Design review of the part built by this model. Coordinates are the model's own, in mm. A direction names the side the tool comes from. Coordinates: 2 decimals unless noted, no trailing zeros. Order: outer loops, then holes, each group sorted by start corner. A loop starts at its lowest first (then second) coordinate and runs counter-clockwise, first axis right, second up.
from build123d import *

# Parameters (mm, degrees)
SKETCH1_W           = 30.2
SKETCH1_H           = 14.75
SKETCH1_W_2         = 25.2
SKETCH1_H_2         = 9.75
BOSS_EXTRUDE1_DEPTH = 20
SKETCH2_W           = 30.2
SKETCH2_H           = 14.75
BOSS_EXTRUDE2_DEPTH = 2.5
SKETCH3_W           = 14.2
SKETCH3_H           = 17.5
CUT_EXTRUDE1_DEPTH  = 2.5
FILLET1_R           = 2.5
FILLET2_R           = 2.5
FILLET3_START       = -8
FILLET3_DEPTH       = 16
FILLET3_START_2     = 4.875
FILLET3_2_DEPTH     = 3.125
FILLET3_3_DEPTH     = 2.5


with BuildPart() as part:
    # Sketch1 → Boss-Extrude1 (new body)
    with BuildSketch(Plane(origin=(0, 0, 0), x_dir=(1, 0, 0), z_dir=(0, 1, 0))):
        Rectangle(SKETCH1_W, SKETCH1_H)
        Rectangle(SKETCH1_W_2, SKETCH1_H_2, mode=Mode.SUBTRACT)
    extrude(amount=BOSS_EXTRUDE1_DEPTH)

    # Sketch2 → Boss-Extrude2 (add)
    with BuildSketch(Plane(origin=(0, 20, 0), x_dir=(1, 0, 0), z_dir=(0, 1, 0))):
        Rectangle(SKETCH2_W, SKETCH2_H)
    extrude(amount=BOSS_EXTRUDE2_DEPTH)

    # Sketch3 → Cut-Extrude1 (cut)
    with BuildSketch(Plane.XY.offset(7.375)):
        with Locations((0, 8.75)):
            Rectangle(SKETCH3_W, SKETCH3_H)
    extrude(amount=-CUT_EXTRUDE1_DEPTH, mode=Mode.SUBTRACT)

    # Fillet1
    fillet1_edges = [part.edges().sort_by_distance(p)[0] for p in [
        (-15.1, 22.5, 0),
        (15.1, 22.5, 0),
    ]]
    fillet(fillet1_edges, radius=FILLET1_R)

    # Fillet2
    fillet2_edges = [part.edges().sort_by_distance(p)[0] for p in [
        (12.6, 20, 0),
        (-12.6, 20, 0),
    ]]
    fillet(fillet2_edges, radius=FILLET2_R)

    # Fillet3: read off the stored shape, not the designer's step
    # Fillet3 outline → Fillet3 (cut)
    with BuildSketch(Plane.XY.offset(FILLET3_START)):
        with BuildLine():
            Line((-15.1, 0), (-12.6, 0))
            ThreePointArc((-12.6, 0), (-14.367766953, 0.732233047), (-15.1, 2.5))
            Line((-15.1, 2.5), (-15.1, 0))
        make_face()
        with BuildLine():
            ThreePointArc((15.1, 2.5), (14.367766953, 0.732233047), (12.6, 0))
            Line((12.6, 0), (15.1, 0))
            Line((15.1, 0), (15.1, 2.5))
        make_face()
    extrude(amount=FILLET3_DEPTH, mode=Mode.SUBTRACT)

    # Fillet3 2 outline → Fillet3 2 (cut)
    with BuildSketch(Plane.XY.offset(FILLET3_START_2)):
        with BuildLine():
            ThreePointArc((-7.1, 2.5), (-7.832233047, 0.732233047), (-9.6, 0))
            Line((-9.6, 0), (-7.1, 0))
            Line((-7.1, 0), (-7.1, 2.5))
        make_face()
        with BuildLine():
            Line((7.1, 2.5), (7.1, 0))
            Line((7.1, 0), (9.6, 0))
            ThreePointArc((9.6, 0), (7.832233047, 0.732233047), (7.1, 2.5))
        make_face()
    extrude(amount=FILLET3_2_DEPTH, mode=Mode.SUBTRACT)

    # Fillet3 3 outline → Fillet3 3 (add)
    with BuildSketch(Plane.XY.offset(FILLET3_START_2)):
        with BuildLine():
            Line((-7.1, 17.5), (-7.1, 15))
            ThreePointArc((-7.1, 15), (-6.367766953, 16.767766953), (-4.6, 17.5))
            Line((-4.6, 17.5), (-7.1, 17.5))
        make_face()
        with BuildLine():
            Line((7.1, 17.5), (4.6, 17.5))
            ThreePointArc((4.6, 17.5), (6.367766953, 16.767766953), (7.1, 15))
            Line((7.1, 15), (7.1, 17.5))
        make_face()
    extrude(amount=FILLET3_3_DEPTH)


solid = part.part
1. Insertion check: pin 1 (4 mm diameter, centred on x = -1.5, z = 1.5, fed in from -Y); pin 2 (1.2 mm diameter, centred on x = 0.5, z = 5.5, fed in from -Y). Each pin has a flat end and moves straight along its axis. Give the tip position at first contact, or say it passes through.
2. To check wall thickness, follow line 1 (Z direction, x = 11.5, y = 10.5) (3 decimals); line 2 (X direction, y = 12.5, z = 2.75); line 3 (Z direction, x = 6, y = 10.5) (3 decimals). State the ranges of each line that lie inside material, in increasing order.
3. Add section D-D (z = 3.5). Give the boundary of the cut face in (x, y).
4. Add section C-C (x = -8.5). Give the boundary of the cut face in (y, z) (3 decimals), and give its area (3 significant figures).
5. Add section A-A (z = 6). Give the boundary of the cut face in (x, y), and give its area (3 significant figures).
6. For faces 4 (the flat face through (0, 11, -7.375)), 5 (the flat face through (12.6, 9, 0)), 6 (the cylindrical face through (-6.387, 16.748, 6.108)), list the 3-axis set-ups (+Z, -Z, +X, -X, +Y, -Y) from which the entire face can be reached by the end or side of a thin tool; tool diameter is ignored.
7. Mouldability with a two-part tool opening along Z and no side actions: class faces 1 (the cylindrical face through (11.887, 19.248, -0.068)), 2 (the flat face through (0, 19, 7.375)), 3 (the cylindrical face through (-14.348, 0.713, -0.103)) as pulls with the +Z half, pulls with the -Z half, needs draft (parallel to the pull), parting line crosses it, or undercut.
8. Add section B-B (y = 14.5). Give the boundary of the cut face in (x, z) (3 decimals), and give its area (3 significant figures).
Solution:
1. pin 1: stops at y = 20
1. pin 2: stops at y = 17.5
2. line 1: z = -7.375 to -4.875, 4.875 to 7.375
2. line 2: x = -15.1 to -12.6, 12.6 to 15.1
2. line 3: z = -7.375 to -4.875
3. outline: (-15.1, 2.5) arc R2.5 ccw to (-12.6, 0) - (-12.6, 17.5) arc R2.5 cw to (-10.1, 20) - (10.1, 20) arc R2.5 cw to (12.6, 17.5) - (12.6, 0) arc R2.5 ccw to (15.1, 2.5) - (15.1, 20) arc R2.5 ccw to (12.6, 22.5) - (-12.6, 22.5) arc R2.5 ccw to (-15.1, 20) - close
4. outline: (0, -7.375) - (22.5, -7.375) - (22.5, 7.375) - (0.255, 7.375) - (0.255, 4.875) - (20, 4.875) - (20, -4.875) - (0, -4.875) - close
4. area: 136 mm2
5. outline: (-15.1, 2.5) arc R2.5 ccw to (-12.6, 0) - (-9.6, 0) arc R2.5 ccw to (-7.1, 2.5) - (-7.1, 15) arc R2.5 cw to (-4.6, 17.5) - (4.6, 17.5) arc R2.5 cw to (7.1, 15) - (7.1, 2.5) arc R2.5 ccw to (9.6, 0) - (12.6, 0) arc R2.5 ccw to (15.1, 2.5) - (15.1, 20) arc R2.5 ccw to (12.6, 22.5) - (-12.6, 22.5) arc R2.5 ccw to (-15.1, 20) - close
5. area: 426 mm2
6. face 4: -Z, +X, -X, +Y, -Y
6. face 5: -Y
6. face 6: +Z, -Y
7. face 1: undercut
7. face 2: pulls with the +Z half
7. face 3: needs draft
8. outline: (-15.1, -7.375) - (15.1, -7.375) - (15.1, 7.375) - (7.1, 7.375) - (7.1, 4.875) - (12.6, 4.875) - (12.6, -4.875) - (-12.6, -4.875) - (-12.6, 4.875) - (-7.1, 4.875) - (-7.1, 7.375) - (-15.1, 7.375) - close
8. area: 164 mm2
